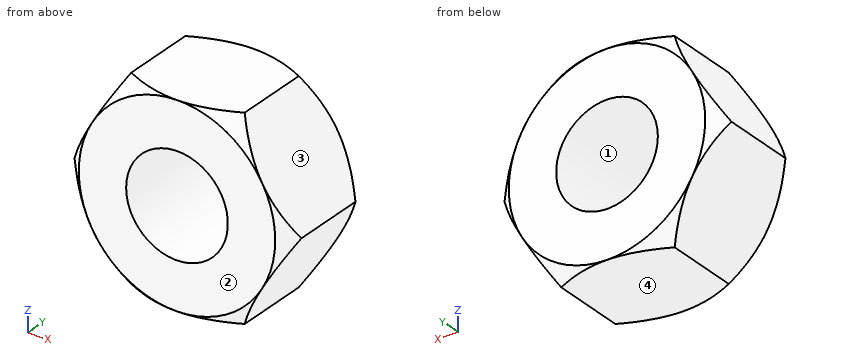
from build123d import *

# Parameters (mm, degrees)
BOSS_EXTRUDE1_DEPTH     = 15
SKETCH2_OUTSIDE_W       = 73.396
SKETCH2_OUTSIDE_H       = 69.064
SKETCH2_OUTSIDE_R       = 14
CUT_EXTRUDE1_DEPTH      = 15
CUT_EXTRUDE1_DRAFT      = -45
MIRROR1_COPY_1_SKETCH_W = 73.396
MIRROR1_COPY_1_SKETCH_H = 69.064
MIRROR1_COPY_1_SKETCH_R = 14
MIRROR1_COPY_1_DEPTH    = 15
MIRROR1_COPY_1_DRAFT    = -45
M16X1_5_TAPPED_HOLE1_D  = 14.5


with BuildPart() as part:
    # Sketch1 → Boss-Extrude1 (new body)
    with BuildSketch(Plane(origin=(0, 0, 0), x_dir=(1, 0, 0), z_dir=(0, 1, 0))):
        Polygon((16.165807537, 0), (8.082903769, 14), (-8.082903769, 14), (-16.165807537, 0), (-8.082903769, -14), (8.082903769, -14), align=None)
    extrude(amount=BOSS_EXTRUDE1_DEPTH)


with BuildPart() as cut_extrude1_tool:
    # Sketch2 outside → Cut-Extrude1 (with draft: the straight prism first)
    with BuildSketch(Plane(origin=(0, 15, 0), x_dir=(1, 0, 0), z_dir=(0, 1, 0))):
        Rectangle(SKETCH2_OUTSIDE_W, SKETCH2_OUTSIDE_H)
        Circle(SKETCH2_OUTSIDE_R, mode=Mode.SUBTRACT)
    extrude(amount=-CUT_EXTRUDE1_DEPTH)
    # Cut-Extrude1: the draft: its side faces are tilted about the plane it starts from
    cut_extrude1_sides = [cut_extrude1_tool.faces().sort_by_distance(p)[0] for p in [
        (0, 7.5, 34.532),
        (36.698, 7.5, 0),
        (0, 7.5, -34.532),
        (-36.698, 7.5, 0),
        (-14, 7.5, 0),
    ]]
    draft(cut_extrude1_sides, Plane(origin=(0, 15, 0), x_dir=(1, 0, 0), z_dir=(0, 1, 0)), CUT_EXTRUDE1_DRAFT)


with BuildPart() as part_1:
    add(part.part)

    # Cut-Extrude1: cut by cut_extrude1_tool
    add(cut_extrude1_tool.part, mode=Mode.SUBTRACT)


with BuildPart() as mirror1_copy_1_tool:
    # Mirror1 copy 1 sketch → Mirror1 copy 1 (with draft: the straight prism first)
    with BuildSketch(Plane.XZ):
        Rectangle(MIRROR1_COPY_1_SKETCH_W, MIRROR1_COPY_1_SKETCH_H)
        Circle(MIRROR1_COPY_1_SKETCH_R, mode=Mode.SUBTRACT)
    extrude(amount=-MIRROR1_COPY_1_DEPTH)
    # Mirror1 copy 1: the draft: its side faces are tilted about the plane it starts from
    mirror1_copy_1_sides = [mirror1_copy_1_tool.faces().sort_by_distance(p)[0] for p in [
        (0, 7.5, 34.532),
        (36.698, 7.5, 0),
        (0, 7.5, -34.532),
        (-36.698, 7.5, 0),
        (-14, 7.5, 0),
    ]]
    draft(mirror1_copy_1_sides, Plane.XZ, MIRROR1_COPY_1_DRAFT)


with BuildPart() as part_2:
    add(part_1.part)

    # Mirror1 copy 1: cut by mirror1_copy_1_tool
    add(mirror1_copy_1_tool.part, mode=Mode.SUBTRACT)

    # M16x1.5 Tapped Hole1 (through all)
    with Locations(Plane(origin=(0, 15, 0), x_dir=(1, 0, 0), z_dir=(0, 1, 0))):
        with Locations((0, 0)):
            Hole(M16X1_5_TAPPED_HOLE1_D / 2)


solid = part_2.part
Input: part model. Units: mm. Frame: model coordinates. Face numbers are marked on the shaded views. Round coordinates to 2 decimals unless told otherwise and drop trailing zeros. Write each loop counter-clockwise with the first axis right and the second up, starting at its lowest first coordinate (ties: lowest second). Pieces come first, ordered by that corner, then holes.
1) Cut plane A-A (y = 10.75). Return the cut outline in (x, z).
2) Draft query along Z for the marked faces 1, 2, 3 and 4. Return one class per face: pulls with the +Z half, pulls with the -Z half, needs draft (parallel to the pull), parting line crosses it, or undercut.
3) Contact query for flat-ended pins moving along their axis: P1, Ø8.5, axis at x = 0, z = 0, coming from the -Y side; P2, Ø6, axis at y = 9, z = 10, coming from the -X side; P3, Ø6, axis at y = 12, z = 6, coming from the -X side; P4, Ø8, axis at y = 6.5, z = 10.5, coming from the -X side. Output: stop coordinate, or through.
4) Ray query, L1, parallel to Z at x = 0, y = 10; L2, parallel to X at y = 4, z = 2.5; L3, parallel to Z at x = -2, y = 2.5. Return the intervals inside material, ascending.
Geometry says:
1. outline: (-16.17, 0) - (-8.08, -14) - (8.08, -14) - (16.17, 0) - (8.08, 14) - (-8.08, 14) - close; hole circle Ø14.5 at (0, 0)
2. face 1: undercut
2. face 2: needs draft
2. face 3: pulls with the +Z half
2. face 4: pulls with the -Z half
3. P1: passes through
3. P2: stops at x = -12.12
3. P3: stops at x = -14.43
3. P4: stops at x = -12.41
4. L1: z = -14 to -7.25, 7.25 to 14
4. L2: x = -14.72 to -6.81, 6.81 to 14.72
4. L3: z = -14 to -6.97, 6.97 to 14
